Check sheet for the drawn part. Datum: minimum x, y, z corner. Units: mm. A direction names the side the tool comes from. Round coordinates to 2 decimals unless told otherwise and drop trailing zeros. Order: outer loops, then holes, each group sorted by start corner. A loop starts at its lowest first (then second) coordinate and runs counter-clockwise, first axis right, second up. Notation, with made-up numbers: (29, 72) -> (56, 72) arc R18 cw to (56, 90) -> close; hole circle Ø1 at (-7.5, 21). An arc over 180 degrees is marked (long way). Write item = value, one per line. Start each with the question number.
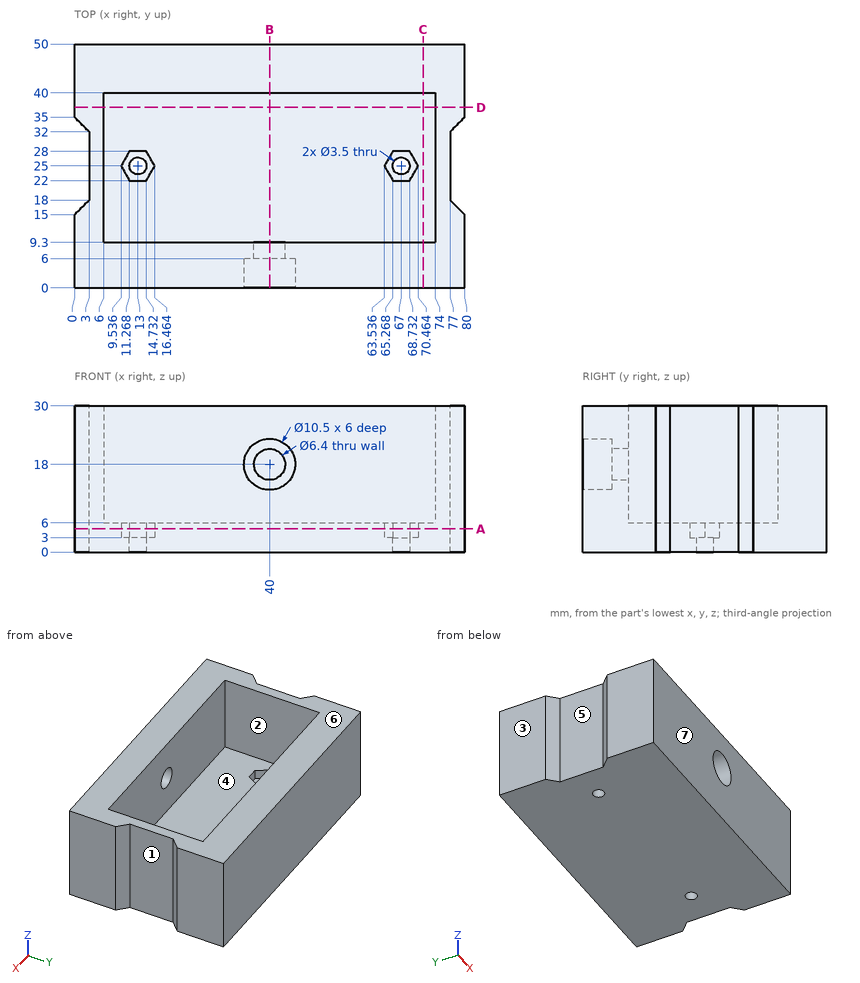
(1) Cross-section at D-D (y = 37). Enter the section's corners in (x, z).
(2) Cross-section at C-C (x = 71.5). Enter the section's corners in (y, z), and give its area (3 significant figures).
(3) Set-up check for the marked faces 1, 2 and 3: record each of +Z, -Z, +X, -X, +Y, -Y from which the full face is reachable in a straight line by a thin tool's end or side.
(4) Cross-section at B-B (x = 40). Enter the section's corners in (y, z), and give its area (3 significant figures).
(5) Scan lines: line 1 along X through (y, z) = (30.5, 10.5); line 2 along Y through (x, z) = (50, 6.5); line 3 along Y through (x, z) = (41.5, 16.75). Record each from-to range of solid material in increasing order. Write a range as from..to.
(6) Depth check by flat-ended pin: pin 1 (15.5 mm diameter, centred on x = 39, y = 23.5, fed in from +Z); pin 2 (1.8 mm diameter, centred on x = 67, y = 25, fed in from +Z); pin 3 (8 mm diameter, centred on y = 11, z = 8, fed in from -X); pin 4 (1.5 mm diameter, centred on x = 43.5, z = 20, fed in from -Y). Enter the tip coordinate at first touch or a pass-through.
(7) Draft check along Y on the marked faces 4, 5, 6 and 7. Enter one of: +Y half, -Y half, draft (parallel to the pull), parting line (faces both ways), or undercut.
(8) Cross-section at A-A (z = 4.75). Give the number of separate pieces and of enclosed holes in the cut face, and give its area (3 significant figures).
Outcome:
q1.outline = (0, 0) -> (80, 0) -> (80, 30) -> (74, 30) -> (74, 6) -> (6, 6) -> (6, 30) -> (0, 30) -> close
q2.outline = (0, 0) -> (50, 0) -> (50, 30) -> (40, 30) -> (40, 6) -> (9.3, 6) -> (9.3, 30) -> (0, 30) -> close
q2.area = 763 mm^2
q3.face_1 = +Z, -Z, +X
q3.face_2 = +Z
q3.face_3 = +Z, -Z, -X, +Y, -Y
q4.outline = (0, 0) -> (50, 0) -> (50, 30) -> (40, 30) -> (40, 6) -> (9.3, 6) -> (9.3, 14.8) -> (6, 14.8) -> (6, 12.75) -> (0, 12.75) -> close; (0, 23.25) -> (6, 23.25) -> (6, 21.2) -> (9.3, 21.2) -> (9.3, 30) -> (0, 30) -> close
q4.area = 679 mm^2
q5.line_1 = 3..6, 74..77
q5.line_2 = 0..9.3, 40..50
q5.line_3 = 40..50
q6.pin_1 = 6
q6.pin_2 = through
q6.pin_3 = 0
q6.pin_4 = 6
q7.face_4 = undercut
q7.face_5 = undercut
q7.face_6 = draft
q7.face_7 = -Y half
q8.separate_pieces = 1
q8.enclosed_holes = 2
q8.area = 3,840 mm^2
